Input: part model. Units: mm. Frame: model coordinates. A direction names the side the tool comes from. Coordinates: 2 decimals unless noted, no trailing zeros. Loops run counter-clockwise (first coordinate to the right, second up) from the corner with the lowest first, then second, coordinate; pieces in that order, holes last.
Item 1: Ray query, line 1 along Y through (x, z) = (-6, 11.25); line 2 along X through (y, z) = (-0.5, 11.5); line 3 along Y through (x, z) = (13.1, 0.55). Return the intervals inside material, ascending.
Item 2: Section A-A on z = 4.5. Return loops of the section in (x, y).
Item 3: Pull-direction query (Z, two-part tool) for faces 1 (the flat face through (0, 11, 19.1)), 2 (the cylindrical face through (21.092, 0.352, 0.493)), 3 (the flat face through (24, -6, 16.1)), 4 (the flat face through (-24.114, 3.164, 17.621)); classes: released by +Z, released by -Z, zero draft, split by the parting line, or undercut.
Item 4: Reachability of faces 5 (the flat face through (-5, -11, 17)), 6 (the flat face through (22, -10, 11)), 7 (the flat face through (-17, -11, 19.1)), 8 (the flat face through (24.114, -3.236, 17.579)), 9 (the flat face through (-25.1, 0, 9)) from +Z, -Z, +X, -X, +Y, -Y: full face, straight path, thin tool, end or side. Return the list, or none.
Item 5: Section C-C on y = 0. Return loops of the section in (x, z).
Item 6: Section B-B on x = -13.1. Return loops of the section in (y, z).
Item 7: Contact query for flat-ended pins moving along their axis: P1, Ø2, axis at x = 22, y = -9.5, coming from the +Z side; P2, Ø1, axis at x = -24, y = -5.5, coming from the +Z side; P3, Ø13, axis at x = 13.1, y = 0, coming from the -Z side; P4, Ø0.8, axis at x = -1.5, y = -11, coming from the +Z side. Output: stop coordinate, or through.
Item 8: Section D-D on x = -2. Return loops of the section in (y, z), and give its area (3 significant figures).
```python
from build123d import *

# Parameters (mm, degrees)
F0_W     = 46.2
F0_H     = 21.3
F1_DEPTH = 19.1
F0_R     = 8
F2_DEPTH = 1
F3_W     = 10
F3_H     = 0.0997345659
F3_H_2   = 3.9002654341
F4_DEPTH = 4
F6_DEPTH = 28
F7_W     = 2
F7_H     = 2
F8_DEPTH = 10


with BuildPart() as f1:
    # F0 (on Top) → F1 (new body)
    with BuildSketch(Plane.XY):
        Polygon((24.1, 11.65), (-24.1, 11.65), (-25.1, 11.65), (-25.1, -11.65), (-24.1, -11.65), (24.4, -11.65), (25.1, -11.65), (25.1, 11.65), align=None)
        Rectangle(F0_W, F0_H, mode=Mode.SUBTRACT)
    extrude(amount=F1_DEPTH)

    # F0 (on Top) → F2 (join)
    with BuildSketch(Plane.XY):
        Rectangle(F0_W, F0_H)
        with Locations((-13.1, 0)):
            Circle(F0_R, mode=Mode.SUBTRACT)
        with BuildLine():
            ThreePointArc((21.1, 0), (13.1, -8), (5.1, 0))
            ThreePointArc((5.1, 0), (13.1, 8), (21.1, 0))
        make_face(mode=Mode.SUBTRACT)
    extrude(amount=F2_DEPTH)

    # F3 (on face) → F4 (cut)
    with BuildSketch(Plane.XZ.offset(11.65)):
        with Locations((0, 19.1498672829)):
            Rectangle(F3_W, F3_H)
        with Locations((0, 17.1498672829)):
            Rectangle(F3_W, F3_H_2)
    extrude(amount=-F4_DEPTH, mode=Mode.SUBTRACT)

    # F5 (on Right) → F6 (cut, symmetric)
    with BuildSketch(Plane.YZ):
        Polygon((9.15, 16.1), (7.15, 19.1), (4.15, 19.1), (2.15, 16.1), align=None)
        Polygon((-2.25, 16.1), (-4.25, 19.1), (-7.25, 19.1), (-9.25, 16.1), align=None)
    extrude(amount=F6_DEPTH, both=True, mode=Mode.SUBTRACT)

    # F7 (on face) → F8 (join)
    with BuildSketch(Plane.XY.offset(1)):
        with Locations((-22.1, 9.65)):
            Rectangle(F7_W, F7_H)
        with Locations((-22.1, -9.65)):
            Rectangle(F7_W, F7_H)
        with Locations((22.1, -9.65)):
            Rectangle(F7_W, F7_H)
        with Locations((22.1, 9.65)):
            Rectangle(F7_W, F7_H)
    extrude(amount=F8_DEPTH)


solid = f1.part
```
Results found:
1. line 1: y = -11.65 to -10.65, 10.65 to 11.65
1. line 2: x = -25.1 to -23.1, 23.1 to 25.1
1. line 3: y = -11.65 to -8, 8 to 11.65
2. outline: (-25.1, -11.65) - (25.1, -11.65) - (25.1, 11.65) - (-25.1, 11.65) - close; hole (-23.1, -8.65) - (-21.1, -8.65) - (-21.1, -10.65) - (21.1, -10.65) - (21.1, -8.65) - (23.1, -8.65) - (23.1, 8.65) - (21.1, 8.65) - (21.1, 10.65) - (-21.1, 10.65) - (-21.1, 8.65) - (-23.1, 8.65) - close
3. face 1: released by +Z
3. face 2: zero draft
3. face 3: undercut
3. face 4: undercut
4. face 5: +Z, -Y
4. face 6: +Z
4. face 7: +Z, +X, -X, +Y, -Y
4. face 8: +X, -X
4. face 9: +Z, -Z, -X, +Y, -Y
5. outline: (-25.1, 0) - (-21.1, 0) - (-21.1, 1) - (-23.1, 1) - (-23.1, 19.1) - (-25.1, 19.1) - close; (-5.1, 0) - (5.1, 0) - (5.1, 1) - (-5.1, 1) - close; (21.1, 0) - (25.1, 0) - (25.1, 19.1) - (23.1, 19.1) - (23.1, 1) - (21.1, 1) - close
6. outline: (-11.65, 0) - (-8, 0) - (-8, 1) - (-10.65, 1) - (-10.65, 19.1) - (-11.65, 19.1) - close; (8, 0) - (11.65, 0) - (11.65, 19.1) - (10.65, 19.1) - (10.65, 1) - (8, 1) - close
7. P1: stops at z = 11
7. P2: stops at z = 16.1
7. P3: passes through
7. P4: stops at z = 15.2
8. outline: (-11.65, 0) - (11.65, 0) - (11.65, 19.1) - (10.65, 19.1) - (10.65, 1) - (-10.65, 1) - (-10.65, 15.2) - (-11.65, 15.2) - close
8. area: 55.6 mm2
